from build123d import *

# Parameters (mm, degrees)
SKETCH1_W             = 100
SKETCH1_H             = 100
BOSS_EXTRUDE1_DEPTH   = 6.35
SKETCH10_W            = 32
SKETCH10_H            = 43.75
BOSS_EXTRUDE2_DEPTH   = 6.35
SKETCH3_R             = 0.99187
CUT_EXTRUDE1_DEPTH    = 107.439583802
M3_CLEARANCE_HOLE1_D  = 3.2
M4_CLEARANCE_HOLE1_D  = 4.3
M3X0_5_TAPPED_HOLE1_D = 2.5
FILLET1_R             = 2


with BuildPart() as part:
    # Sketch1 → Boss-Extrude1 (new body)
    with BuildSketch(Plane(origin=(0, 0, 0), x_dir=(1, 0, 0), z_dir=(0, 1, 0))):
        Rectangle(SKETCH1_W, SKETCH1_H)
    extrude(amount=BOSS_EXTRUDE1_DEPTH)

    # Sketch10 → Boss-Extrude2 (add)
    with BuildSketch(Plane(origin=(0, 6.35, 0), x_dir=(1, 0, 0), z_dir=(0, 1, 0))):
        with Locations((0, 71.875)):
            Rectangle(SKETCH10_W, SKETCH10_H)
    extrude(amount=-BOSS_EXTRUDE2_DEPTH)

    # Sketch3 → Cut-Extrude1 (cut, through all)
    with BuildSketch(Plane(origin=(0, 6.35, 0), x_dir=(1, 0, 0), z_dir=(0, 1, 0))):
        with Locations(Location((-36, 0, 0), (0, 0, 270))):
            Circle(SKETCH3_R)
        with Locations(Location((36, 0, 0), (0, 0, 270))):
            Circle(SKETCH3_R)
    extrude(amount=-CUT_EXTRUDE1_DEPTH, mode=Mode.SUBTRACT)

    # M3 Clearance Hole1 (through all)
    with Locations(Plane(origin=(0, 6.35, 0), x_dir=(1, 0, 0), z_dir=(0, 1, 0))):
        with Locations((-47.5, 45.5), (47.5, 45.5), (47.5, -45.5), (-47.5, -45.5), (-31.176914536, -18), (31.176914536, -18), (18, 31.176914536), (-18, 31.176914536)):
            Hole(M3_CLEARANCE_HOLE1_D / 2)

    # M4 Clearance Hole1 (through all)
    with Locations(Plane(origin=(0, 6.35, 0), x_dir=(1, 0, 0), z_dir=(0, 1, 0))):
        with Locations((-35.355, -35.355), (-35.355, 35.355), (35.355, 35.355), (35.355, -35.355)):
            Hole(M4_CLEARANCE_HOLE1_D / 2)

    # M3x0.5 Tapped Hole1 (through all)
    with Locations(Plane(origin=(0, 6.35, 0), x_dir=(1, 0, 0), z_dir=(0, 1, 0))):
        with Locations((-13, 89.5), (13, 89.5), (13, 61), (-13, 61)):
            Hole(M3X0_5_TAPPED_HOLE1_D / 2)

    # Fillet1
    fillet1_edges = [part.edges().sort_by_distance(p)[0] for p in [
        (16, 3.175, -93.75),
        (-16, 3.175, -93.75),
        (-16, 3.175, -50),
        (16, 3.175, -50),
        (50, 3.175, 50),
        (-50, 3.175, 50),
        (-50, 3.175, -50),
        (50, 3.175, -50),
    ]]
    fillet(fillet1_edges, radius=FILLET1_R)


solid = part.part
Can you work these out from the model? Positions are in its coordinate system, mm. A direction names the side the tool comes from. Give positions to 0.01 mm unless a question says otherwise; leave off trailing zeros. Loops run counter-clockwise (first coordinate to the right, second up) from the corner with the lowest first, then second, coordinate; pieces in that order, holes last. Notation, with made-up numbers: (-27, 50) - (7, 50) arc R22 ccw to (7, 71) - close; hole circle Ø10 at (12, 41). An arc over 180 degrees is marked (long way). Return JSON: item names as keys, results as strings.
1. I want a section at B-B on y = 2. Give the number of separate pieces and of enclosed holes in the cut face, and give its area (3 significant figures).
Output values:
{"separate pieces": "1", "enclosed holes": "18", "area": "11,200 mm²"}
2. We'd pull the mould along Z, two halves only. Please class faces 1 (the face through (-1, 6.35, -7)), 2 (the face through (33, 3, -50)), 3 (the face through (-48.24, 3.13, -44.08)), 4 (the face through (-36.51, 3.13, 33.54)): +Z half, -Z half, draft (parallel to the pull), parting line (faces both ways), or undercut.
Output values:
{"face 1": "draft", "face 2": "-Z half", "face 3": "undercut", "face 4": "undercut"}
3. For faces 5 (the face through (-48.24, 3.13, 46.92)), 6 (the face through (-33, 3, -50)), which set-ups out of +Z, -Z, +X, -X, +Y, -Y let a thin tool reach every point of the face, with its end or its side?
Output values:
{"face 5": "+Y, -Y", "face 6": "-Z, -X, +Y, -Y"}
4. If I drill on line 1 (Z direction, x = -47.5, y = 3.25); line 2 (X direction, y = 2, z = -89.5); line 3 (X direction, y = 2.5, z = 45.5), over which ranges is the centre line in solid material (lowest first)?
Output values:
{"line 1": "z = -50 to -47.1, -43.9 to 43.9, 47.1 to 50", "line 2": "x = -16 to -14.25, -11.75 to 11.75, 14.25 to 16", "line 3": "x = -50 to -49.1, -45.9 to 45.9, 49.1 to 50"}
5. I want a section at C-C on z = -66. Please give me the cut outline in (x, y), and give its area (3 significant figures).
Output values:
{"outline": "(-16, 0) - (16, 0) - (16, 6.35) - (-16, 6.35) - close", "area": "203 mm²"}
6. I want a section at A-A on z = 18. Please give me the cut outline in (x, y), and give its area (3 significant figures).
Output values:
{"outline": "(-50, 0) - (-32.78, 0) - (-32.78, 6.35) - (-50, 6.35) - close; (-29.58, 0) - (29.58, 0) - (29.58, 6.35) - (-29.58, 6.35) - close; (32.78, 0) - (50, 0) - (50, 6.35) - (32.78, 6.35) - close", "area": "594 mm²"}
7. I'm going to push flat-ended pins straight in: pin 1 Ø6 at (x, z) = (22.5, -6.5) entering from -Y; pin 2 Ø1.5 at (x, z) = (13, -61) entering from +Y; pin 3 Ø1 at (x, y) = (-33, 3) entering from -Z; pin 4 Ø3 at (y, z) = (2, -63) entering from -X. Where does each tip first touch, or does it pass through?
Output values:
{"pin 1": "stops at y = 0", "pin 2": "passes through", "pin 3": "stops at z = -50", "pin 4": "stops at x = -16"}
